Part model, mm, in its own coordinate system. A direction names the side the tool comes from. Give positions to 0.01 mm unless a question says otherwise; leave off trailing zeros. Write each loop counter-clockwise with the first axis right and the second up, starting at its lowest first coordinate (ties: lowest second). Pieces come first, ordered by that corner, then holes. Notation, with made-up numbers: M 29.5,-28.75 L 35.5,-28.75 A16 ccw 35.5,-11.75 Z; hole C 47,72 d3. An arc over 180 degrees is marked long. Use CSV: the item, a comma, the result in double quotes. Start each with the question number.
1. Band-saw the part on C-C, the plane y = 1.95. List the corners of the cut face in (x, z) (3 decimals), then the cut area to 3 significant figures.
2. 3-axis set-ups, long thin cutter, end or side, ignore diameter. For faces 1 (the face through (2.286, 2, -19)), 2 (the face through (0, 2, 58.623)): which of +Z, -Z, +X, -X, +Y, -Y reach the whole face in a straight line?
3. Band-saw the part on B-B, the plane x = -3.81. List the corners of the cut face in (y, z).
4. Band-saw the part on A-A, the plane z = -9.5. List the corners of the cut face in (x, y) (1 decimal).
5. Mould opens along X. For faces 3 (the face through (15.875, 2, 1)), 4 (the face through (10, 0, -1)), 5 (the face through (0, 2, -21.463)) say: pulls with the +X half, pulls with the -X half, needs draft (parallel to the pull), parting line crosses it, or undercut.
6. Drill centre lines: line 1 along X through (y, z) = (2.8, -3.5) (3 decimals); line 2 along Z through (x, y) = (6, 0.35); line 3 along X through (y, z) = (1.65, 21) (1 decimal). Where is each one in solid material? Low to high. Write a range as from..to.
from build123d import *

# Parameters (mm, degrees)
SKETCH1_W           = 31.75
SKETCH1_H           = 117.2464
BOSS_EXTRUDE1_DEPTH = 4.7625
SKETCH3_W           = 15.24
SKETCH3_H           = 35.814
CUT_EXTRUDE1_DEPTH  = 4.7625
SKETCH4_R           = 1.905
CUT_EXTRUDE9_DEPTH  = 4.7625


with BuildPart() as part:
    # Sketch1 → Boss-Extrude1 (new body)
    with BuildSketch(Plane(origin=(0, 0, 0), x_dir=(1, 0, 0), z_dir=(0, 1, 0))):
        Rectangle(SKETCH1_W, SKETCH1_H)
    extrude(amount=BOSS_EXTRUDE1_DEPTH)

    # Sketch3 → Cut-Extrude1 (cut)
    with BuildSketch(Plane(origin=(0, 4.7625, 0), x_dir=(1, 0, 0), z_dir=(0, 1, 0))):
        Rectangle(SKETCH3_W, SKETCH3_H)
    extrude(amount=-CUT_EXTRUDE1_DEPTH, mode=Mode.SUBTRACT)

    # Sketch4 → Cut-Extrude9 (cut)
    with BuildSketch(Plane(origin=(0, 4.7625, 0), x_dir=(1, 0, 0), z_dir=(0, 1, 0))):
        with Locations(Location((-3.81, -21.209, 0), (0, 0, 270))):
            Circle(SKETCH4_R)
        with BuildLine():
            Line((-2.286, 21.463), (-2.286, 17.907))
            Line((-2.286, 17.907), (2.286, 17.907))
            Line((2.286, 17.907), (2.286, 20.066))
            ThreePointArc((2.286, 20.066), (1.966546058, 20.728684934), (1.922009269, 21.463))
            Line((1.922009269, 21.463), (-2.286, 21.463))
        make_face()
        with BuildLine():
            ThreePointArc((1.922009269, 21.463), (1.966546058, 20.728684934), (2.286, 20.066))
            Line((2.286, 20.066), (2.286, 21.463))
            Line((2.286, 21.463), (1.922009269, 21.463))
        make_face()
        with BuildLine():
            Line((2.286, 21.463), (2.286, 20.066))
            ThreePointArc((2.286, 20.066), (4.412413894, 19.401758317), (5.715, 21.209))
            ThreePointArc((5.715, 21.209), (3.937284441, 23.109742926), (1.922009269, 21.463))
            Line((1.922009269, 21.463), (2.286, 21.463))
        make_face()
    extrude(amount=-CUT_EXTRUDE9_DEPTH, mode=Mode.SUBTRACT)


solid = part.part
Output:
1,outline,"M -15.875,-58.623 L 15.875,-58.623 L 15.875,58.623 L -15.875,58.623 Z; hole M -7.62,-17.907 L -2.286,-17.907 L -2.286,-21.463 L 1.922,-21.463 A1.905 ccw long 2.286,-20.066 L 2.286,-17.907 L 7.62,-17.907 L 7.62,17.907 L -7.62,17.907 Z; hole C -3.81,21.209 d3.81"
1,area,"3,140 mm²"
2,face 1,"+Y, -Y"
2,face 2,"+Z, +X, -X, +Y, -Y"
3,outline,"M 0,-58.62 L 4.76,-58.62 L 4.76,-17.91 L 0,-17.91 Z; M 0,17.91 L 4.76,17.91 L 4.76,19.3 L 0,19.3 Z; M 0,23.11 L 4.76,23.11 L 4.76,58.62 L 0,58.62 Z"
4,outline,"M -15.9,0 L -7.6,0 L -7.6,4.8 L -15.9,4.8 Z; M 7.6,0 L 15.9,0 L 15.9,4.8 L 7.6,4.8 Z"
5,face 3,"pulls with the +X half"
5,face 4,"needs draft"
5,face 5,"undercut"
6,line 1,"x = -15.875..-7.62, 7.62..15.875"
6,line 2,"z = -58.62..-17.91, 17.91..58.62"
6,line 3,"x = -15.9..-5.7, -1.9..15.9"
